Design review of the part shown in the three views and the two pictorial views. Dimensions are in mm from the part's minimum x, y and z. A direction names the side the tool comes from. Give positions to 0.01 mm unless a question says otherwise; leave off trailing zeros. Loops run counter-clockwise (first coordinate to the right, second up) from the corner with the lowest first, then second, coordinate; pieces in that order, holes last.
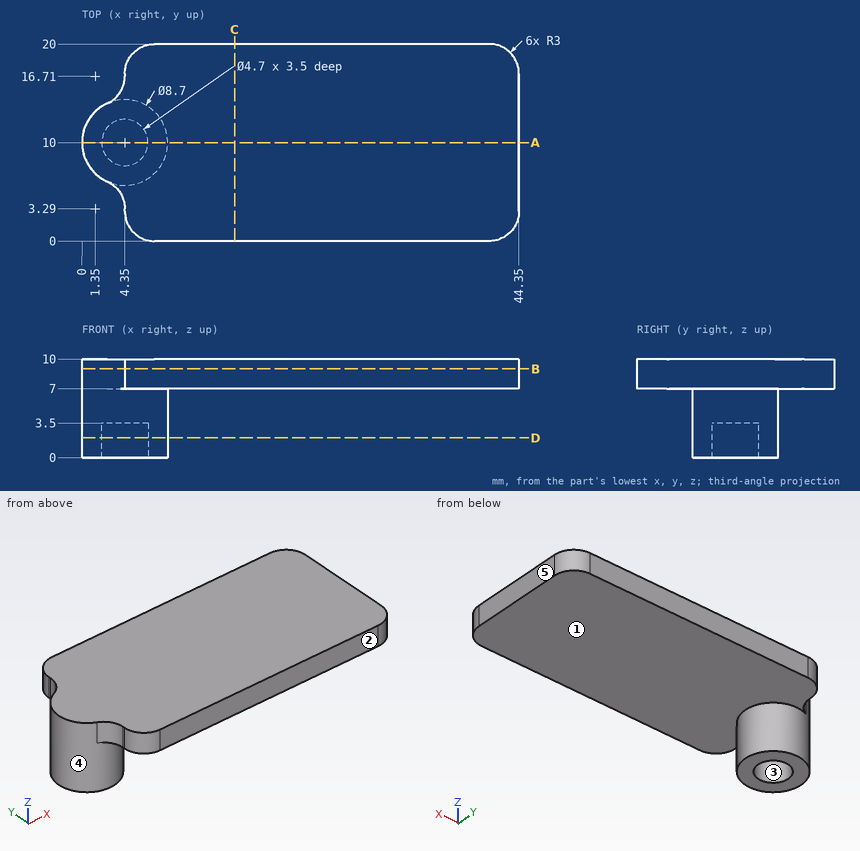
Q1. Draft analysis for pull direction Y (two halves, no side actions). For the marked faces 1, 2 and 3, state which applies: pulls with the +Y half, pulls with the -Y half, needs draft (parallel to the pull), parting line crosses it, or undercut.
Results:
face 1: needs draft
face 2: pulls with the -Y half
face 3: undercut
Q2. Tool access review of the marked faces 4 and 5: name each direction out of +Z, -Z, +X, -X, +Y, -Y from which nothing blocks a thin tool from reaching the whole face with its end or side.
Results:
face 4: -Z
face 5: +Z, -Z, +X, +Y, -Y
Q3. Wall thickness on line 1 (Y direction, x = 4.35, z = 1.1); line 2 (Z direction, x = 20, y = 7.25); line 3 (X direction, y = 8.25, z = 2): over which ranges is each line inside the solid? List them lowest first.
Results:
line 1: y = 5.65 to 7.65, 12.35 to 14.35
line 2: z = 7 to 10
line 3: x = 0.37 to 2.78, 5.92 to 8.33
Q4. Insertion check: pin 1 (10 mm diameter, centred on x = 27, y = 10, fed in from -Z); pin 2 (6 mm diameter, centred on y = 15.5, z = 3, fed in from -X). Each pin has a flat end and moves straight along its axis. Give the tip position at first contact, or say it passes through.
Results:
pin 1: stops at z = 7
pin 2: stops at x = 0.79
Q5. Take a section at B-B (z = 9). Give the boundary of the cut face in (x, y).
Results:
outline: (2.57, 6.03) arc R3 cw to (4.35, 3.29) - (4.35, 3) arc R3 ccw to (7.35, 0) - (41.35, 0) arc R3 ccw to (44.35, 3) - (44.35, 17) arc R3 ccw to (41.35, 20) - (7.35, 20) arc R3 ccw to (4.35, 17) - (4.35, 16.71) arc R3 cw to (2.57, 13.97) arc R4.35 ccw to start
Q6. Take a section at C-C (x = 15.5). Give the boundary of the cut face in (y, z).
Results:
outline: (0, 7) - (20, 7) - (20, 10) - (0, 10) - close
Q7. Take a section at A-A (y = 10). Give the boundary of the cut face in (x, z).
Results:
outline: (0, 0) - (2, 0) - (2, 3.5) - (6.7, 3.5) - (6.7, 0) - (8.7, 0) - (8.7, 7) - (44.35, 7) - (44.35, 10) - (0, 10) - close
Q8. Take a section at D-D (z = 2). Give the boundary of the cut face in (x, y).
Results:
outline: circle Ø8.7 at (4.35, 10); hole circle Ø4.7 at (4.35, 10)
